Input: part model. Units: mm. Frame: model coordinates. Round coordinates to 2 decimals unless told otherwise and drop trailing zeros. Loops run counter-clockwise (first coordinate to the right, second up) from the corner with the lowest first, then second, coordinate; pieces in that order, holes last.
(1) Cut plane D-D, the plane y = -20. Output: boundary loops of the cut face in (x, z), and give its area (3 significant figures).
(2) Line query: line 1 (Y direction, x = 58.5, z = 2.2); line 2 (Y direction, x = -38, z = 0.7); line 3 (Y direction, x = 15.5, z = 2.95). Output: solid intervals per line, ascending.
(3) Cut plane A-A, the plane x = 0. Output: boundary loops of the cut face in (y, z), and give its area (3 significant figures).
(4) First-contact query: pin 1 Ø2 at (x, y) = (59.22, -46.85) entering from -Z. Flat tip, straight axial feed; report the tip coordinate or a pass-through.
(5) Cut plane B-B, the plane y = 84. Output: boundary loops of the cut face in (x, z), and give its area (3 significant figures).
(6) Cut plane C-C, the plane z = 1.65. Give the number of separate pieces and of enclosed holes in the cut face, and give its area (3 significant figures).
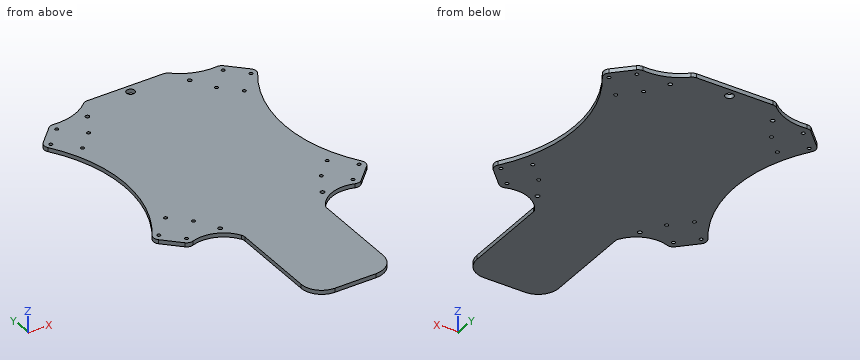
from build123d import *

# Parameters (mm, degrees)
SKETCH2_R           = 1.5
SKETCH2_R_2         = 3
BOSS_EXTRUDE1_DEPTH = 3
SKETCH3_R           = 1.25
F_45_DEGREES_DEPTH  = 188.565988388
FILLET1_R           = 5
FILLET2_R           = 5
FILLET3_R           = 5
FILLET4_R           = 5
FILLET5_R           = 5
FILLET6_R           = 5
FILLET7_R           = 5
FILLET8_R           = 5
FILLET10_R          = 5
FILLET11_R          = 5
FILLET12_R          = 5
FILLET13_R          = 5


with BuildPart() as part:
    # Sketch2 → Boss-Extrude1 (new body)
    with BuildSketch(Plane.XY):
        with BuildLine():
            Line((-79.195959493, 62.225396744), (-62.225396744, 79.195959493))
            ThreePointArc((-62.225396744, 79.195959493), (-44.806778225, 80.702789346), (-30, 90))
            Line((-30, 90), (30, 90))
            ThreePointArc((30, 90), (44.806778225, 80.702789346), (62.225396744, 79.195959493))
            Line((62.225396744, 79.195959493), (79.195959493, 62.225396744))
            ThreePointArc((79.195959493, 62.225396744), (58.781303002, 0), (79.195959493, -62.225396744))
            Line((79.195959493, -62.225396744), (62.225396744, -79.195959493))
            ThreePointArc((62.225396744, -79.195959493), (43.875108319, -77.923881554), (30, -90))
            Line((30, -90), (30, -155))
            ThreePointArc((30, -155), (25.606601718, -165.606601718), (15, -170))
            Line((15, -170), (-15, -170))
            ThreePointArc((-15, -170), (-25.606601718, -165.606601718), (-30, -155))
            Line((-30, -155), (-30, -90))
            ThreePointArc((-30, -90), (-43.875108319, -77.923881554), (-62.225396744, -79.195959493))
            Line((-62.225396744, -79.195959493), (-79.195959493, -62.225396744))
            ThreePointArc((-79.195959493, -62.225396744), (-58.781303002, 0), (-79.195959493, 62.225396744))
        make_face()
        with Locations((-37.5, 75)):
            Circle(SKETCH2_R, mode=Mode.SUBTRACT)
        with Locations((37.5, 75)):
            Circle(SKETCH2_R, mode=Mode.SUBTRACT)
        with Locations((37.5, -75)):
            Circle(SKETCH2_R, mode=Mode.SUBTRACT)
        with Locations((-37.5, -75)):
            Circle(SKETCH2_R, mode=Mode.SUBTRACT)
        with Locations((0, 84)):
            Circle(SKETCH2_R_2, mode=Mode.SUBTRACT)
    extrude(amount=BOSS_EXTRUDE1_DEPTH)

    # Sketch3 → 45 Degrees (cut, through all)
    with BuildSketch(Plane.XY.offset(3)):
        with Locations((-73.362328548, 60.987959877)):
            Circle(SKETCH3_R)
        with Locations((-59.220192924, 46.845824254)):
            Circle(SKETCH3_R)
        with Locations(Location((-60.987959877, 73.362328548, 0), (0, 0, 180))):
            Circle(SKETCH3_R)
        with Locations(Location((-46.845824254, 59.220192924, 0), (0, 0, 180))):
            Circle(SKETCH3_R)
        with Locations(Location((59.220192924, 46.845824254, 0), (0, 0, 180))):
            Circle(SKETCH3_R)
        with Locations(Location((73.362328548, 60.987959877, 0), (0, 0, 180))):
            Circle(SKETCH3_R)
        with Locations((60.987959877, 73.362328548)):
            Circle(SKETCH3_R)
        with Locations((46.845824254, 59.220192924)):
            Circle(SKETCH3_R)
        with Locations(Location((-59.220192924, -46.845824254, 0), (0, 0, 180))):
            Circle(SKETCH3_R)
        with Locations((-46.845824254, -59.220192924)):
            Circle(SKETCH3_R)
        with Locations((-60.987959877, -73.362328548)):
            Circle(SKETCH3_R)
        with Locations(Location((-73.362328548, -60.987959877, 0), (0, 0, 180))):
            Circle(SKETCH3_R)
        with Locations((59.220192924, -46.845824254)):
            Circle(SKETCH3_R)
        with Locations((73.362328548, -60.987959877)):
            Circle(SKETCH3_R)
        with Locations(Location((60.987959877, -73.362328548, 0), (0, 0, 180))):
            Circle(SKETCH3_R)
        with Locations(Location((46.845824254, -59.220192924, 0), (0, 0, 180))):
            Circle(SKETCH3_R)
    extrude(amount=-F_45_DEGREES_DEPTH, mode=Mode.SUBTRACT)

    # Fillet1
    fillet1_edges = [part.edges().sort_by_distance(p)[0] for p in [
        (-30, 90, 1.5),
    ]]
    fillet(fillet1_edges, radius=FILLET1_R)

    # Fillet2
    fillet2_edges = [part.edges().sort_by_distance(p)[0] for p in [
        (-79.195959493, 62.225396744, 1.5),
    ]]
    fillet(fillet2_edges, radius=FILLET2_R)

    # Fillet3
    fillet3_edges = [part.edges().sort_by_distance(p)[0] for p in [
        (-62.225396744, 79.195959493, 1.5),
    ]]
    fillet(fillet3_edges, radius=FILLET3_R)

    # Fillet4
    fillet4_edges = [part.edges().sort_by_distance(p)[0] for p in [
        (62.225396744, 79.195959493, 1.5),
    ]]
    fillet(fillet4_edges, radius=FILLET4_R)

    # Fillet5
    fillet5_edges = [part.edges().sort_by_distance(p)[0] for p in [
        (30, 90, 1.5),
    ]]
    fillet(fillet5_edges, radius=FILLET5_R)

    # Fillet6
    fillet6_edges = [part.edges().sort_by_distance(p)[0] for p in [
        (79.195959493, 62.225396744, 1.5),
    ]]
    fillet(fillet6_edges, radius=FILLET6_R)

    # Fillet7
    fillet7_edges = [part.edges().sort_by_distance(p)[0] for p in [
        (79.195959493, -62.225396744, 1.5),
    ]]
    fillet(fillet7_edges, radius=FILLET7_R)

    # Fillet8
    fillet8_edges = [part.edges().sort_by_distance(p)[0] for p in [
        (62.225396744, -79.195959493, 1.5),
    ]]
    fillet(fillet8_edges, radius=FILLET8_R)

    # Fillet10
    fillet10_edges = [part.edges().sort_by_distance(p)[0] for p in [
        (30, -90, 1.5),
    ]]
    fillet(fillet10_edges, radius=FILLET10_R)

    # Fillet11
    fillet11_edges = [part.edges().sort_by_distance(p)[0] for p in [
        (-30, -90, 1.5),
    ]]
    fillet(fillet11_edges, radius=FILLET11_R)

    # Fillet12
    fillet12_edges = [part.edges().sort_by_distance(p)[0] for p in [
        (-79.195959493, -62.225396744, 1.5),
    ]]
    fillet(fillet12_edges, radius=FILLET12_R)

    # Fillet13
    fillet13_edges = [part.edges().sort_by_distance(p)[0] for p in [
        (-62.225396744, -79.195959493, 1.5),
    ]]
    fillet(fillet13_edges, radius=FILLET13_R)


solid = part.part
Reported:
1. outline: (-60.7, 0) - (60.7, 0) - (60.7, 3) - (-60.7, 3) - close
1. area: 364 mm2
2. line 1: y = -77.71 to -47.87, -45.82 to 45.82, 47.87 to 78.82
2. line 2: y = -80.84 to -76.41, -73.59 to 73.59, 76.41 to 83.78
2. line 3: y = -169.99 to 90
3. outline: (-170, 0) - (81, 0) - (81, 3) - (-170, 3) - close; (87, 0) - (90, 0) - (90, 3) - (87, 3) - close
3. area: 762 mm2
4. pin 1: passes through
5. outline: (-37.62, 0) - (-3, 0) - (-3, 3) - (-37.62, 3) - close; (3, 0) - (37.62, 0) - (37.62, 3) - (3, 3) - close
5. area: 208 mm2
6. separate pieces: 1
6. enclosed holes: 21
6. area: 27,100 mm2
